Source: three-view drawing plus pictorial views. Frame: mm from the lowest corner of the part. Coordinates: 2 decimals unless noted, no trailing zeros. Write each loop counter-clockwise with the first axis right and the second up, starting at its lowest first coordinate (ties: lowest second). Pieces come first, ordered by that corner, then holes. Notation, with made-up numbers: M -28,32 L 30,32 A24 ccw 30,50 Z; hole C 2.5,55.5 d5. An arc over 180 degrees is marked long. Use CSV: the item, a comma, the result in double quotes.
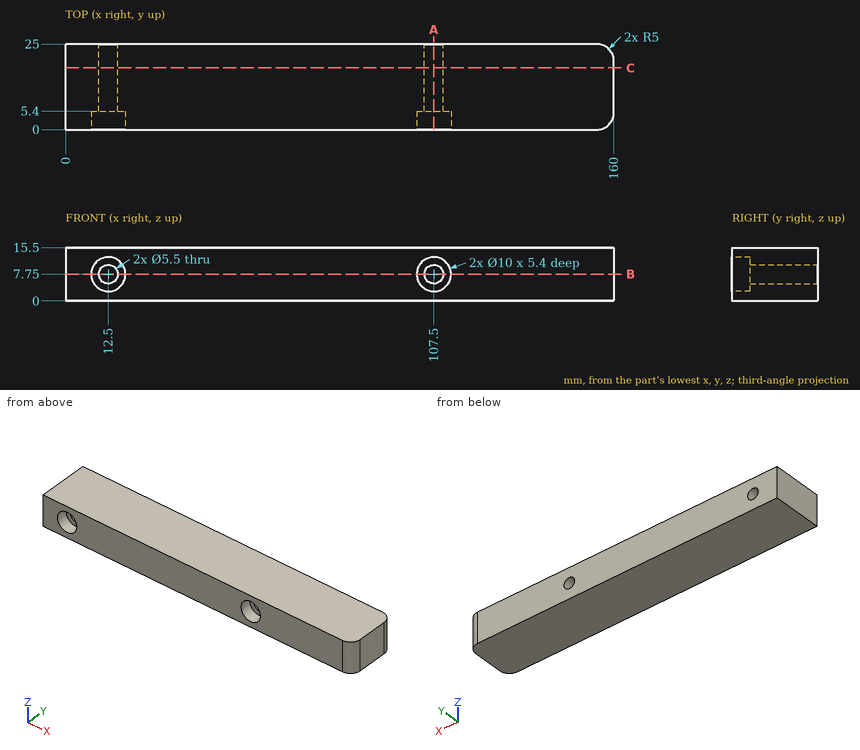
1. Material intervals for line 1 (Z direction, x = 12.5, y = 15.25); line 2 (X direction, y = 15.5, z = 10); line 3 (X direction, y = 9.75, z = 10.25), sorted ascending. Write a range as [from, to].
Resolved:
line 1,"z = [0, 5], [10.5, 15.5]"
line 2,"x = [0, 10.92], [14.08, 105.92], [109.08, 160]"
line 3,"x = [0, 11.35], [13.65, 106.35], [108.65, 160]"
2. Contact query for flat-ended pins moving along their axis: pin 1 Ø9 at (x, z) = (12.5, 7.75) entering from -Y; pin 2 Ø5 at (x, z) = (107.5, 7.75) entering from -Y; pin 3 Ø3 at (y, z) = (3, 12) entering from +X. Output: stop coordinate, or through.
Resolved:
pin 1,"stops at y = 5.4"
pin 2,"passes through"
pin 3,"stops at x = 159.97"
3. Section A-A (x = 107.5). Return loops of the section in (y, z).
Resolved:
outline,"M 0,0 L 25,0 L 25,5 L 5.4,5 L 5.4,2.75 L 0,2.75 Z; M 0,12.75 L 5.4,12.75 L 5.4,10.5 L 25,10.5 L 25,15.5 L 0,15.5 Z"
4. Section B-B (z = 7.75). Return loops of the section in (x, y).
Resolved:
outline,"M 0,0 L 7.5,0 L 7.5,5.4 L 9.75,5.4 L 9.75,25 L 0,25 Z; M 15.25,5.4 L 17.5,5.4 L 17.5,0 L 102.5,0 L 102.5,5.4 L 104.75,5.4 L 104.75,25 L 15.25,25 Z; M 110.25,5.4 L 112.5,5.4 L 112.5,0 L 155,0 A5 ccw 160,5 L 160,20 A5 ccw 155,25 L 110.25,25 Z"
5. Section C-C (y = 18). Return loops of the section in (x, z), then the cut area to 3 significant figures.
Resolved:
outline,"M 0,0 L 160,0 L 160,15.5 L 0,15.5 Z; hole C 12.5,7.75 d5.5; hole C 107.5,7.75 d5.5"
area,"2,430 mm^2"
